Autodesk Inventor part; units mm, degrees
ref_plane "YZ Plane" through (0, 0, 0) normal (1, 0, 0) x (0, 1, 0)
ref_plane "XZ Plane" through (0, 0, 0) normal (0, 1, 0) x (-1, 0, 0)
ref_plane "XY Plane" through (0, 0, 0) normal (0, 0, 1) x (1, 0, 0)
sketch "Sketch1" plane through (0, 0, 0) normal (0, 1, 0) x (-1, 0, 0)
  line L0 (15, 0) -> (15, -15)
  line L1 (15, -15) -> (0, -15)
  line L2 (0, -15) -> (0, -12)
  line L3 (0, -12) -> (12, -12)
  line L4 (12, -12) -> (12, 0)
  line L5 (12, 0) -> (15, 0)
  point P0 (0, 0)
  dimension "d0" = 15
  dimension "d1" = 15
  dimension "d10" = 3
  dimension "d11" = 12
  dimension "d12" = 12
extrude "Extrusion1" add sketch "Sketch1" along normal blind 86
sketch "Sketch4" plane through (-12, 0, 0) normal (1, 0, 0) x (0, 0, -1)
  line L0 (0, 0) -> (0, 86)
  line L1 (12, 0) -> (12, 86)
  line L2 (0, 86) -> (12, 86)
  line L3 (12, 86) -> (12, 83)
  line L4 (12, 83) -> (0, 83)
  line L5 (0, 83) -> (0, 86)
  dimension "d13" = 3
extrude "Extrusion3" add sketch "Sketch4" along normal blind 3
sketch "Sketch6" plane through (-12, 0, -12) normal (0, 0, 1) x (1, 0, 0)
  line L0 (3, 86) -> (12, 86)
  line L1 (12, 86) -> (3, 86)
  line L2 (3, 86) -> (3, 83)
  line L3 (3, 83) -> (12, 83)
  line L4 (12, 83) -> (12, 86)
  point P0 (12, 0)
extrude "Extrusion4" add sketch "Sketch6" along normal blind 12
fillet "Fillet3" radius 2 7 edges at (-7.5, 86, -15) (-15, 86, -7.5) (-15, 43, -15) (0, 43, -15) (-7.5, 86, 0) (0, 86, -7.5) (-15, 43, 0)
properties part number "DoosjeHoeken" material "ABS Plastic"
Geometry check sheet. Reference: the model listing, model coordinates, mm. A direction names the side the tool comes from. Give positions to 0.01 mm unless a question says otherwise; leave off trailing zeros. Write each loop counter-clockwise with the first axis right and the second up, starting at its lowest first coordinate (ties: lowest second). Pieces come first, ordered by that corner, then holes. Notation, with made-up numbers: M 66.5,56 L 93.5,56 A19 ccw 93.5,72 Z; hole C 8.25,66 d9. An arc over 180 degrees is marked long. Answer as CSV lines item,"result". Start each with the question number.
Q1. Tool access check on faces 1 (the face through (-6, 83, -6)), 2 (the face through (-14.43, 85.4, -7.58)). Record the directions out of +Z, -Z, +X, -X, +Y, -Y that give a thin tool (end or side, any length) a straight path to the whole face; none if there is none.
Q2. Section check A-A, the plane z = -7. Record the cut outline in (x, y), then the cut area to 3 significant figures.
Q3. Material ranges on L1, parallel to Y at x = -10.5, z = -3.75; L2, parallel to X at y = 22.5, z = -4, recorded low to high.
Q4. Section check C-C, the plane y = 71.5. Record the cut outline in (x, z), then the cut area to 3 significant figures.
Q5. Section check B-B, the plane x = -3.75. Record the cut outline in (y, z).
Q6. Go/stop test with a flat-tipped pin: pin 1 (4 mm diameter, centred on x = -3, y = 20, fed in from +Z). Record where the tip stops, or that it passes through.
Geometry says:
1,face 1,"+Z, +X, -Y"
1,face 2,"+Z, -Z, -X, +Y"
2,outline,"M -15,0 L -12,0 L -12,83 L 0,83 L 0,84 A2 ccw -2,86 L -13,86 A2 ccw -15,84 Z"
2,area,"292 mm^2"
3,L1,"83 to 86"
3,L2,"-15 to -12"
4,outline,"M -15,-13 A2 ccw -13,-15 L -2,-15 A2 ccw 0,-13 L 0,-12 L -12,-12 L -12,0 L -13,0 A2 ccw -15,-2 Z"
4,area,"78.4 mm^2"
5,outline,"M 0,-15 L 84,-15 A2 ccw 86,-13 L 86,-2 A2 ccw 84,0 L 83,0 L 83,-12 L 0,-12 Z"
6,pin 1,"z = -12"
